Could you check a few things on this model? Use its own coordinates, in mm. A direction names the side the tool comes from. Round coordinates to 2 decimals unless told otherwise and drop trailing zeros. Order: outer loops, then holes, each group sorted by start corner. A loop starts at its lowest first (then second) coordinate and runs counter-clockwise, first axis right, second up. Notation, with made-up numbers: (68.25, 32) - (84.25, 32) arc R18 ccw to (84.25, 51) - close; hole circle Ø8 at (10.25, 16.25). An arc over 180 degrees is marked (long way). Return JSON: item names as keys, results as strings. Group by question number.
Solid Edge part; units mm, degrees
sketch "Sketch1" plane through (0, 0, 0) normal (0, 0, 1) x (1, 0, 0)
  circle A0 centre (0, 0) radius 60
  circle A1 centre (0, 0) radius 20
extrude "Protrusion1" add sketch "Sketch1" along normal blind 76
sketch "Sketch2" plane through (0, 0, 76) normal (0, 0, 1) x (1, 0, 0)
  circle A0 centre (0, 0) radius 20
  circle A1 centre (0, 0) radius 33
extrude "ExtrudedProtrusion_2" add sketch "Sketch2" along normal blind 8.7
sketch "Sketch3" plane through (0, 0, 0) normal (0, 0, -1) x (1, 0, 0)
  circle A0 centre (0, 0) radius 20
  circle A1 centre (0, 0) radius 28.75
extrude "ExtrudedProtrusion_3" add sketch "Sketch3" along normal blind 9.5
properties material "Aluminum, 6061-T6"
1) I want a section at C-C, the plane z = 53. List the corners of the cut face in (x, y) for me, plus the area to 3 significant figures.
2) Will these pins go through, and if not, where does the flat tip stop? pin 1 (10 mm diameter, centred on y = 35.5, z = 42, fed in from -X); pin 2 (8 mm diameter, centred on y = 43.5, z = 41.5, fed in from -X); pin 3 (6 mm diameter, centred on x = 33.5, z = 71, fed in from +Y).
3) If I drill on line 1 along Y through (x, z) = (0, 29); line 2 along Z through (x, y) = (-0.5, 32.5); line 3 along Z through (x, y) = (48, -24.5), over which ranges is the centre line in solid material (lowest first)? Write a range as from..to.
4) We'd pull the mould along X, two halves only. Please class faces 1 (the cylindrical face through (-4.336, -19.524, 38.259)), 2 (the cylindrical face through (-6.232, -28.066, -4.684)), 3 (the flat face through (26, -26, 76)): +X half, -X half, draft (parallel to the pull), parting line (faces both ways), or undercut.
5) I want a section at A-A, the plane y = 0. List the corners of the cut face in (x, z) for me, plus the area to 3 significant figures.
6) I want a section at D-D, the plane y = 24.5. List the corners of the cut face in (x, z) for me, plus the area to 3 significant figures.
7) For faces 4 (the flat face through (26, 14, 0)), 5 (the cylindrical face through (30.5, 12.6, 80.3)), 6 (the flat face through (-6, 20, -9.5)), which set-ups out of +Z, -Z, +X, -X, +Y, -Y let a thin tool reach every point of the face, with its end or its side?
8) I want a section at B-B, the plane x = 3.5. List the corners of the cut face in (y, z) for me.
Outcome:
{
 "1": {"outline": "circle Ø120 at (0, 0); hole circle Ø40 at (0, 0)", "area": "10,100 mm^2"},
 "2": {"pin 1": "x = -51.67", "pin 2": "x = -45.16", "pin 3": "y = 51.67"},
 "3": {"line 1": "-60..-20, 20..60", "line 2": "0..84.7", "line 3": "0..76"},
 "4": {"face 1": "undercut", "face 2": "parting line", "face 3": "draft"},
 "5": {"outline": "(-60, 0) - (-28.75, 0) - (-28.75, -9.5) - (-20, -9.5) - (-20, 84.7) - (-33, 84.7) - (-33, 76) - (-60, 76) - close; (20, -9.5) - (28.75, -9.5) - (28.75, 0) - (60, 0) - (60, 76) - (33, 76) - (33, 84.7) - (20, 84.7) - close", "area": "6,470 mm^2"},
 "6": {"outline": "(-54.77, 0) - (-15.04, 0) - (-15.04, -9.5) - (15.04, -9.5) - (15.04, 0) - (54.77, 0) - (54.77, 76) - (22.11, 76) - (22.11, 84.7) - (-22.11, 84.7) - (-22.11, 76) - (-54.77, 76) - close", "area": "9,000 mm^2"},
 "7": {"face 4": "-Z", "face 5": "+Z", "face 6": "-Z, +X, -X, +Y, -Y"},
 "8": {"outline": "(-59.9, 0) - (-28.54, 0) - (-28.54, -9.5) - (-19.69, -9.5) - (-19.69, 84.7) - (-32.81, 84.7) - (-32.81, 76) - (-59.9, 76) - close; (19.69, -9.5) - (28.54, -9.5) - (28.54, 0) - (59.9, 0) - (59.9, 76) - (32.81, 76) - (32.81, 84.7) - (19.69, 84.7) - close"}
}
